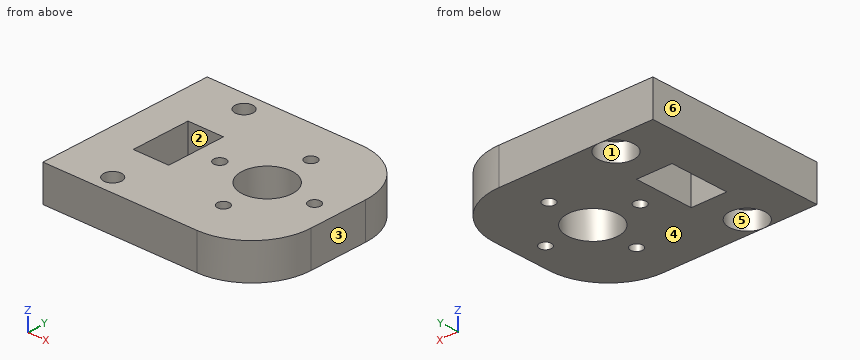
```python
from build123d import *

# Parameters (mm, degrees)
ESQUISSE1_W             = 50
ESQUISSE1_H             = 30
BOSS_EXTRU_1_DEPTH      = 6
ESQUISSE4_W             = 5
ESQUISSE4_H             = 30
ENL_V_MAT_EXTRU_2_DEPTH = 6
ESQUISSE6_R             = 1.5
ENL_V_MAT_EXTRU_3_DEPTH = 6
ESQUISSE7_R             = 2.995
ENL_V_MAT_EXTRU_4_DEPTH = 3
ESQUISSE8_W             = 6
ESQUISSE8_H             = 10
ENL_V_MAT_EXTRU_5_DEPTH = 6
ESQUISSE10_R            = 1.005
ENL_V_MAT_EXTRU_6_DEPTH = 6
ESQUISSE11_R            = 4.25
ENL_V_MAT_EXTRU_7_DEPTH = 6
ESQUISSE12_W            = 9
ESQUISSE12_H            = 30
ENL_V_MAT_EXTRU_8_DEPTH = 6
CONG_1_R                = 10


with BuildPart() as part:
    # Esquisse1 → Boss.-Extru.1 (new body)
    with BuildSketch(Plane.XY):
        with Locations((0.584677419, -1.784274194)):
            Rectangle(ESQUISSE1_W, ESQUISSE1_H)
    extrude(amount=BOSS_EXTRU_1_DEPTH)

    # Esquisse4 → Enlèv. mat.-Extru.2 (cut)
    with BuildSketch(Plane.XY.offset(6)):
        with Locations((-21.915322581, -1.784274194)):
            Rectangle(ESQUISSE4_W, ESQUISSE4_H)
    extrude(amount=-ENL_V_MAT_EXTRU_2_DEPTH, mode=Mode.SUBTRACT)

    # Esquisse6 → Enlèv. mat.-Extru.3 (cut)
    with BuildSketch(Plane(origin=(0, 0, 0), x_dir=(-1, 0, 0), z_dir=(0, 0, -1))):
        with Locations((10.415322581, 10.215725806)):
            Circle(ESQUISSE6_R)
        with Locations((10.415322581, -13.784274194)):
            Circle(ESQUISSE6_R)
    extrude(amount=-ENL_V_MAT_EXTRU_3_DEPTH, mode=Mode.SUBTRACT)

    # Esquisse7 → Enlèv. mat.-Extru.4 (cut)
    with BuildSketch(Plane(origin=(0, 0, 0), x_dir=(-1, 0, 0), z_dir=(0, 0, -1))):
        with Locations((10.415322581, -13.784274194)):
            Circle(ESQUISSE7_R)
        with Locations((10.415322581, 10.215725806)):
            Circle(ESQUISSE7_R)
    extrude(amount=-ENL_V_MAT_EXTRU_4_DEPTH, mode=Mode.SUBTRACT)

    # Esquisse8 → Enlèv. mat.-Extru.5 (cut)
    with BuildSketch(Plane(origin=(0, 0, 0), x_dir=(-1, 0, 0), z_dir=(0, 0, -1))):
        with Locations((10.415322581, -1.784274194)):
            Rectangle(ESQUISSE8_W, ESQUISSE8_H)
    extrude(amount=-ENL_V_MAT_EXTRU_5_DEPTH, mode=Mode.SUBTRACT)

    # Esquisse10 → Enlèv. mat.-Extru.6 (cut)
    with BuildSketch(Plane(origin=(0, 0, 0), x_dir=(-1, 0, 0), z_dir=(0, 0, -1))):
        with Locations((-4.584677419, 6.215725806)):
            Circle(ESQUISSE10_R)
        with Locations((-12.584677419, -1.784274194)):
            Circle(ESQUISSE10_R)
        with Locations((3.415322581, -1.784274194)):
            Circle(ESQUISSE10_R)
        with Locations((-4.584677419, -9.784274194)):
            Circle(ESQUISSE10_R)
    extrude(amount=-ENL_V_MAT_EXTRU_6_DEPTH, mode=Mode.SUBTRACT)

    # Esquisse11 → Enlèv. mat.-Extru.7 (cut)
    with BuildSketch(Plane(origin=(0, 0, 0), x_dir=(-1, 0, 0), z_dir=(0, 0, -1))):
        with Locations((-4.584677419, -1.784274194)):
            Circle(ESQUISSE11_R)
    extrude(amount=-ENL_V_MAT_EXTRU_7_DEPTH, mode=Mode.SUBTRACT)

    # Esquisse12 → Enlèv. mat.-Extru.8 (cut)
    with BuildSketch(Plane(origin=(0, 0, 0), x_dir=(-1, 0, 0), z_dir=(0, 0, -1))):
        with Locations((-21.084677419, -1.784274194)):
            Rectangle(ESQUISSE12_W, ESQUISSE12_H)
    extrude(amount=-ENL_V_MAT_EXTRU_8_DEPTH, mode=Mode.SUBTRACT)

    # Congé1
    cong_1_edges = [part.edges().sort_by_distance(p)[0] for p in [
        (16.584677419, 13.215725806, 3),
        (16.584677419, -16.784274194, 3),
    ]]
    fillet(cong_1_edges, radius=CONG_1_R)


solid = part.part
```
Verification items for the finished model (mm, model axes). Face numbers are marked on the shaded views. A direction names the side the tool comes from. Coordinates: 2 decimals unless noted, no trailing zeros. Order: outer loops, then holes, each group sorted by start corner. A loop starts at its lowest first (then second) coordinate and runs counter-clockwise, first axis right, second up. Notation, with made-up numbers: (26.5, 63.25) -> (63.5, 63.25) arc R27 ccw to (63.5, 86.25) -> close; hole circle Ø1 at (-34.75, 62.25). An arc over 180 degrees is marked (long way). Put each result on its own line as item: value. Start each with the question number.
1) Cross-section at D-D (y = -4.25). Enter the section's corners in (x, z).
2) Material ranges on L1, parallel to X at y = -2.25, z = 4.8; L2, parallel to X at y = -0.5, z = 3.45; L3, parallel to Y at x = -4, z = 3.1, recorded low to high.
3) Go/stop test with flat-tipped pins: pin 1 (5.5 mm diameter, centred on x = -10.42, y = 10.22, fed in from -Z); pin 2 (1.6 mm diameter, centred on x = 4.58, y = 6.22, fed in from -Z). Record where each tip stops, or that it passes through.
4) Tool access check on the marked faces 1, 2 and 3. Record the directions out of +Z, -Z, +X, -X, +Y, -Y that give a thin tool (end or side, any length) a straight path to the whole face; none if there is none.
5) Cross-section at B-B (x = -9.5). Enter the section's corners in (y, z).
6) Release check for a two-part mould opening along X. For the marked faces 4, 5 and 6 record: pulls with the +X half, pulls with the -X half, needs draft (parallel to the pull), parting line crosses it, or undercut.
7) Cross-section at A-A (y = -13.25). Enter the section's corners in (x, z).
8) Cross-section at C-C (z = 5). State how many separate pieces and enclosed holes the cut face has, plus the area to 3 significant figures.
Geometry check:
1. outline: (-19.42, 0) -> (-13.42, 0) -> (-13.42, 6) -> (-19.42, 6) -> close; (-7.42, 0) -> (1.12, 0) -> (1.12, 6) -> (-7.42, 6) -> close; (8.05, 0) -> (16.58, 0) -> (16.58, 6) -> (8.05, 6) -> close
2. L1: x = -19.42 to -13.42, -7.42 to -4.31, -2.52 to 0.36, 8.81 to 11.69, 13.48 to 16.58
2. L2: x = -19.42 to -13.42, -7.42 to 0.53, 8.64 to 16.58
2. L3: y = -16.78 to -2.6, -0.97 to 13.22
3. pin 1: stops at z = 3
3. pin 2: passes through
4. face 1: -Z
4. face 2: +Z, -Z
4. face 3: +Z, -Z, +X, +Y, -Y
5. outline: (-16.78, 0) -> (-16.64, 0) -> (-16.64, 3) -> (-14.97, 3) -> (-14.97, 6) -> (-16.78, 6) -> close; (-12.6, 3) -> (-10.93, 3) -> (-10.93, 0) -> (-6.78, 0) -> (-6.78, 6) -> (-12.6, 6) -> close; (3.22, 0) -> (7.36, 0) -> (7.36, 3) -> (9.03, 3) -> (9.03, 6) -> (3.22, 6) -> close; (11.4, 3) -> (13.07, 3) -> (13.07, 0) -> (13.22, 0) -> (13.22, 6) -> (11.4, 6) -> close
6. face 4: needs draft
6. face 5: undercut
6. face 6: pulls with the -X half
7. outline: (-19.42, 0) -> (-13.36, 0) -> (-13.36, 3) -> (-11.82, 3) -> (-11.82, 6) -> (-19.42, 6) -> close; (-9.01, 3) -> (-7.47, 3) -> (-7.47, 0) -> (14.21, 0) -> (14.21, 6) -> (-9.01, 6) -> close
8. separate pieces: 1
8. enclosed holes: 8
8. area: 894 mm^2
